Geometry: see drawing. Coordinates: mm, zero at the bounding-box minimum. A direction names the side the tool comes from. Coordinates: 2 decimals unless noted, no trailing zeros. Loops run counter-clockwise (first coordinate to the right, second up) from the corner with the lowest first, then second, coordinate; pieces in that order, holes last.
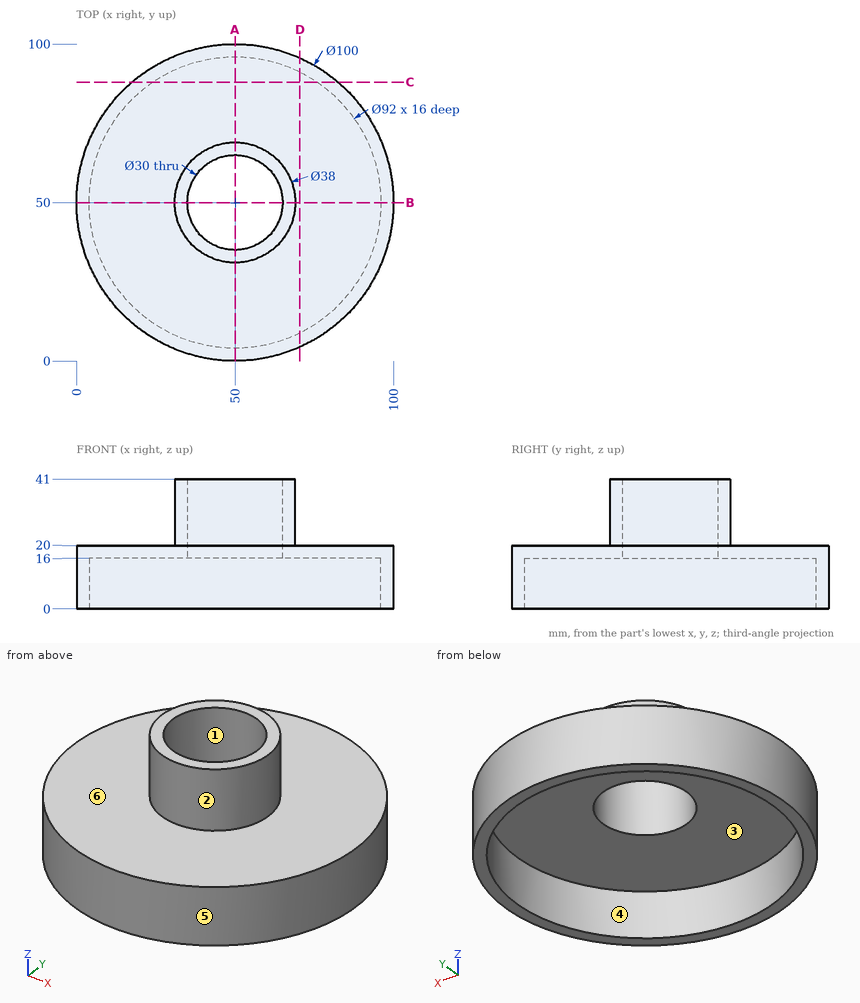
Item 1: Section query C-C (y = 88). Output: boundary loops of the cut face in (x, z).
Result:
outline: (17.5, 0) - (24.08, 0) - (24.08, 16) - (75.92, 16) - (75.92, 0) - (82.5, 0) - (82.5, 20) - (17.5, 20) - close
Item 2: Mould query, pull axis X, two halves, no side actions, for the marked faces 4, 5 and 6. Classes: +X half, -X half, draft (parallel to the pull), parting line (faces both ways), or undercut.
Result:
face 4: undercut
face 5: parting line
face 6: draft
Item 3: Line query: L1, parallel to Y at x = 50, z = 22.75; L2, parallel to X at y = 50, z = 8. Output: solid intervals per line, ascending.
Result:
L1: y = 31 to 35, 65 to 69
L2: x = 0 to 4, 96 to 100
Item 4: Reachability of the marked faces 1, 2 and 3 from +Z, -Z, +X, -X, +Y, -Y: full face, straight path, thin tool, end or side. Return the list, or none.
Result:
face 1: +Z, -Z
face 2: +Z
face 3: -Z
Item 5: Section query D-D (x = 70.5). Output: boundary loops of the cut face in (y, z).
Result:
outline: (4.4, 0) - (8.82, 0) - (8.82, 16) - (91.18, 16) - (91.18, 0) - (95.6, 0) - (95.6, 20) - (4.4, 20) - close
Item 6: Section query A-A (x = 50). Output: boundary loops of the cut face in (y, z).
Result:
outline: (0, 0) - (4, 0) - (4, 16) - (35, 16) - (35, 41) - (31, 41) - (31, 20) - (0, 20) - close; (65, 16) - (96, 16) - (96, 0) - (100, 0) - (100, 20) - (69, 20) - (69, 41) - (65, 41) - close
Item 7: Contact query for flat-ended pins moving along their axis: P1, Ø10, axis at x = 44, z = 26.5, coming from the +Y side; P2, Ø12, axis at x = 22.5, y = 25.5, coming from the +Z side; P3, Ø1.5, axis at x = 71, z = 8, coming from the -Y side. Output: stop coordinate, or through.
Result:
P1: stops at y = 68.97
P2: stops at z = 20
P3: stops at y = 4.28
